from build123d import *

# Parameters (mm, degrees)
SKETCH_1_R               = 46.5
EXTRUDE_1_DEPTH          = 15
SKETCH_2_R               = 31.5
CUT_EXTRUDE_1_DEPTH      = 6.5
SKETCH_3_R               = 3.25
CUT_EXTRUDE_2_DEPTH      = 9.5
PATTERN_CIRCULAR_1_COUNT = 4
SKETCH_4_R               = 5.5
CUT_EXTRUDE_3_DEPTH      = 6.2
SKETCH_5_R               = 2.75
CUT_EXTRUDE_4_DEPTH      = 16
PATTERN_CIRCULAR_2_COUNT = 4
SKETCH_6_R               = 4.75
CUT_EXTRUDE_5_DEPTH      = 5.5
PATTERN_CIRCULAR_3_COUNT = 4


with BuildPart() as part:
    # 草图1 → 凸台-拉伸1 (new body)
    with BuildSketch(Plane(origin=(0, 0, 0), x_dir=(0, 0, -1), z_dir=(1, 0, 0))):
        Circle(SKETCH_1_R)
    extrude(amount=EXTRUDE_1_DEPTH)

    # 草图2 → 切除-拉伸1 (cut)
    with BuildSketch(Plane(origin=(15, 0, 0), x_dir=(0, 0, -1), z_dir=(1, 0, 0))):
        Circle(SKETCH_2_R)
    extrude(amount=-CUT_EXTRUDE_1_DEPTH, mode=Mode.SUBTRACT)

    # 草图3 → 切除-拉伸2 (cut, through all)
    with BuildSketch(Plane(origin=(8.5, 0, 0), x_dir=(0, 0, -1), z_dir=(1, 0, 0))):
        with Locations((0, 25)):
            Circle(SKETCH_3_R)
    cut_extrude_2 = extrude(amount=-CUT_EXTRUDE_2_DEPTH, mode=Mode.SUBTRACT)

    # 阵列(圆周)1: 切除-拉伸2 ×4 about axis
    pattern_circular_1_axis = Axis((0, 0, 0), (1, 0, 0))
    for i in range(1, PATTERN_CIRCULAR_1_COUNT):
        add(cut_extrude_2.rotate(pattern_circular_1_axis, i * 360 / PATTERN_CIRCULAR_1_COUNT), mode=Mode.SUBTRACT)

    # 草图4 → 切除-拉伸3 (cut)
    with BuildSketch(Plane.ZY):
        with Locations((0, 25)):
            Circle(SKETCH_4_R)
        with Locations((-25, 0)):
            Circle(SKETCH_4_R)
        with Locations((0, -25)):
            Circle(SKETCH_4_R)
        with Locations((25, 0)):
            Circle(SKETCH_4_R)
    extrude(amount=-CUT_EXTRUDE_3_DEPTH, mode=Mode.SUBTRACT)

    # 草图5 → 切除-拉伸4 (cut, through all)
    with BuildSketch(Plane(origin=(15, 0, 0), x_dir=(0, 0, -1), z_dir=(1, 0, 0))):
        with Locations((41, 0)):
            Circle(SKETCH_5_R)
    cut_extrude_4 = extrude(amount=-CUT_EXTRUDE_4_DEPTH, mode=Mode.SUBTRACT)

    # 阵列(圆周)2: 切除-拉伸4 ×4 about axis
    pattern_circular_2_axis = Axis((0, 0, 0), (1, 0, 0))
    for i in range(1, PATTERN_CIRCULAR_2_COUNT):
        add(cut_extrude_4.rotate(pattern_circular_2_axis, i * 360 / PATTERN_CIRCULAR_2_COUNT), mode=Mode.SUBTRACT)

    # 草图6 → 切除-拉伸5 (cut)
    with BuildSketch(Plane(origin=(15, 0, 0), x_dir=(0, 0, -1), z_dir=(1, 0, 0))):
        with Locations((0, -41)):
            Circle(SKETCH_6_R)
    cut_extrude_5 = extrude(amount=-CUT_EXTRUDE_5_DEPTH, mode=Mode.SUBTRACT)

    # 阵列(圆周)3: 切除-拉伸5 ×4 about axis
    pattern_circular_3_axis = Axis((0, 0, 0), (1, 0, 0))
    for i in range(1, PATTERN_CIRCULAR_3_COUNT):
        add(cut_extrude_5.rotate(pattern_circular_3_axis, i * 360 / PATTERN_CIRCULAR_3_COUNT), mode=Mode.SUBTRACT)


solid = part.part
Geometry check sheet. Reference: the model listing, model coordinates, mm. A direction names the side the tool comes from. Give positions to 0.01 mm unless a question says otherwise; leave off trailing zeros. Loops run counter-clockwise (first coordinate to the right, second up) from the corner with the lowest first, then second, coordinate; pieces in that order, holes last. Notation, with made-up numbers: M -5,8.25 L -1,8.25 A13 cw -1,28.25 Z; hole C 45.5,-9 d3. An arc over 180 degrees is marked long. Write each question's results on one line, items separated by ' | '.
1) Section check D-D, the plane z = 9. Record the boundary of the cut face in (x, y), plus the area to 3 significant figures.
Answers follow:
outline: M 0,-45.62 L 15,-45.62 L 15,-30.19 L 8.5,-30.19 L 8.5,30.19 L 15,30.19 L 15,45.62 L 0,45.62 Z | area: 976 mm2
2) Section check A-A, the plane z = 25. Record the boundary of the cut face in (x, y), plus the area to 3 significant figures.
Answers follow:
outline: M 0,-39.21 L 15,-39.21 L 15,-19.16 L 8.5,-19.16 L 8.5,-3.25 L 6.2,-3.25 L 6.2,-5.5 L 0,-5.5 Z; M 0,5.5 L 6.2,5.5 L 6.2,3.25 L 8.5,3.25 L 8.5,19.16 L 15,19.16 L 15,39.21 L 0,39.21 Z | area: 844 mm2
3) Release check for a two-part mould opening along Y. For faces 1 (the face through (7.366, 21.827, 0.705)), 2 (the face through (7.4, 13.97, -44.35)), 3 (the face through (0, 1, 1)) record: +Y half, -Y half, draft (parallel to the pull), parting line (faces both ways), or undercut.
Answers follow:
face 1: undercut | face 2: parting line | face 3: draft
4) Thickness scan on line 1 (Y direction, x = 2.25, z = -5); line 2 (Y direction, x = 13, z = -3); line 3 (Z direction, x = 3, y = 41). Record the ranges inside material, lowest first.
Answers follow:
line 1: -46.23 to -27.29, -22.71 to 22.71, 27.29 to 46.23 | line 2: -46.4 to -44.68, -37.32 to -31.36, 31.36 to 37.32, 44.68 to 46.4 | line 3: -21.94 to -2.75, 2.75 to 21.94
5) Gauge pin test, flat ends, axial feed: pin 1 (2 mm diameter, centred on x = 6.5, z = 22, fed in from -Y); pin 2 (4 mm diameter, centred on y = 0, z = 25, fed in from +X); pin 3 (7 mm diameter, centred on y = 0, z = -41, fed in from +X); pin 4 (5 mm diameter, centred on x = 8.5, z = -21.5, fed in from -Y). Record the tip position at first contact, or that the pin passes through.
Answers follow:
pin 1: y = -41.49 | pin 2: through | pin 3: x = 9.5 | pin 4: y = -42.44
6) Tool access check on faces 4 (the face through (12.29, -36.29, 0.62)), 5 (the face through (3.06, 28.72, -4.05)), 6 (the face through (4.817, -38.253, -0.121)). Record the directions out of +Z, -Z, +X, -X, +Y, -Y that give a thin tool (end or side, any length) a straight path to the whole face; none if there is none.
Answers follow:
face 4: +X | face 5: -X | face 6: +X, -X
7) Section check B-B, the plane x = 11. Record the boundary of the cut face in (y, z).
Answers follow:
outline: C 0,0 d93; hole C -41,0 d9.5; hole C 0,0 d63; hole C 0,-41 d9.5; hole C 0,41 d9.5; hole C 41,0 d9.5
